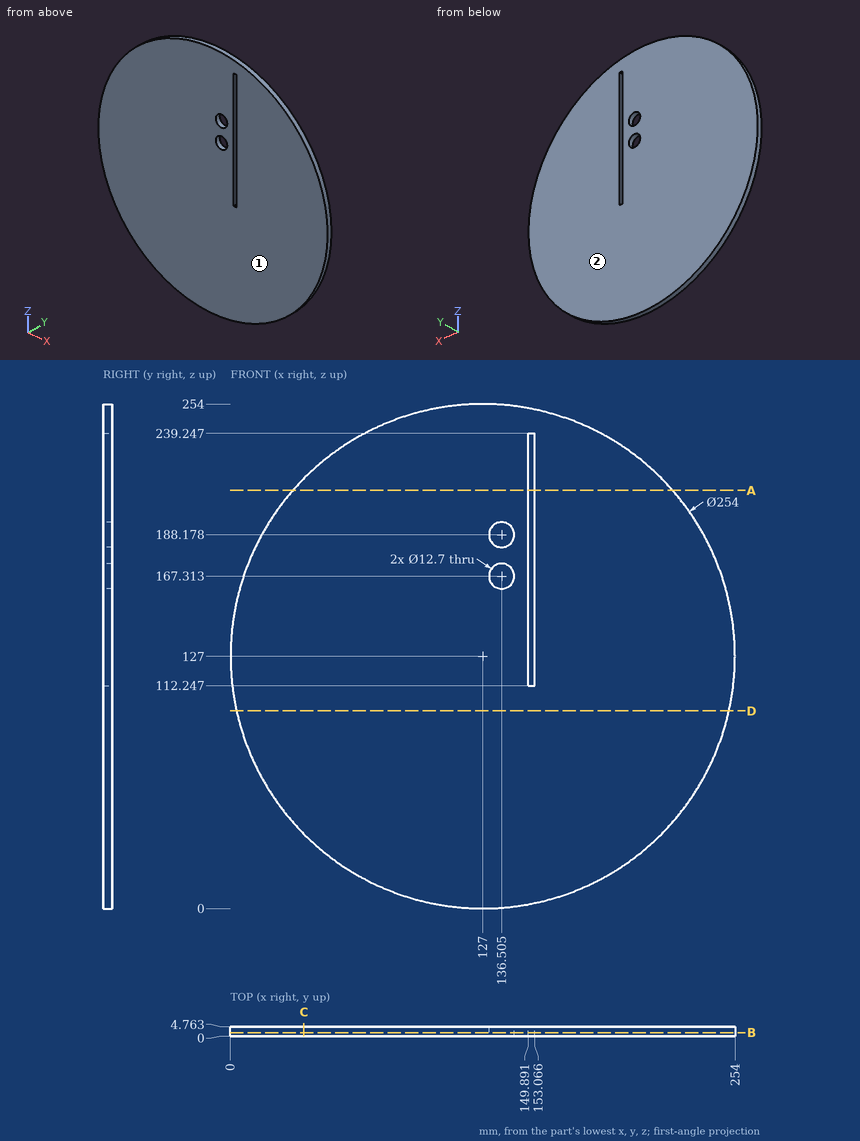
Could you check a few things on this drawing? It's one solid part, dimensions in mm from its lowest x, y, z. Coordinates: 2 decimals unless noted, no trailing zeros. Write each loop counter-clockwise with the first axis right and the second up, starting at its lowest first coordinate (ties: lowest second). Pieces come first, ordered by that corner, then holes. Notation, with made-up numbers: M 72.5,-29 L 96.5,-29 A13 ccw 96.5,-20 Z; hole C 12,-39.5 d2. An arc over 180 degrees is marked long. One line per question, with ' | ' between items.
1) Imagine slicing it at A-A, the plane z = 210.5. Write out the boundary of the cut face in (x, y).
Checks:
outline: M 31.31,0 L 149.89,0 L 149.89,4.76 L 31.31,4.76 Z; M 153.07,0 L 222.69,0 L 222.69,4.76 L 153.07,4.76 Z
2) Imagine slicing it at C-C, the plane x = 37. Write out the boundary of the cut face in (y, z) (1 decimal).
Checks:
outline: M 0,37.4 L 4.8,37.4 L 4.8,216.6 L 0,216.6 Z
3) Imagine slicing it at B-B, the plane y = 1.65. Give the number of separate pieces and of enclosed holes in the cut face, and give its area (3 significant figures).
Checks:
separate pieces: 1 | enclosed holes: 3 | area: 50,000 mm²
4) For pin 1 Ø1 at (x, y) = (152, 1.5) entering from -Z (1 decimal); pin 2 Ø2.5 at (y, z) = (1.5, 150.5) entering from +X (1 decimal); pin 3 Ø2.5 at (x, y) = (152, 3) entering from +Z, each with a flat end and sliding along its axis, tell me the tip position at first contact or that it passes through.
Checks:
pin 1: z = 2.4 | pin 2: x = 252 | pin 3: z = 251.76
5) If we mould it in two halves opening along Y, with no side actions, what happens to the marked faces 1 and 2? For each: released by +Y, released by -Y, zero draft, split by the parting line, or undercut.
Checks:
face 1: released by -Y | face 2: released by +Y
6) Imagine slicing it at D-D, the plane z = 99.5. Write out the boundary of the cut face in (x, y), and give its area (3 significant figures).
Checks:
outline: M 3.01,0 L 250.99,0 L 250.99,4.76 L 3.01,4.76 Z | area: 1,180 mm²
7) I need wall thicknesses on probe 1 along X at (y, z) = (0.2, 194) (1 decimal); probe 2 along Z at (x, y) = (135, 2.5) (1 decimal); probe 3 along X at (y, z) = (4.5, 168.5) (1 decimal). Which ranges of each line are inside material? Lowest first, please. Write a range as [from, to].
Checks:
probe 1: [19.1, 134], [139, 149.9], [153.1, 234.9] | probe 2: [0.3, 161.1], [173.5, 182], [194.3, 253.7] | probe 3: [7, 130.3], [142.7, 149.9], [153.1, 247]
